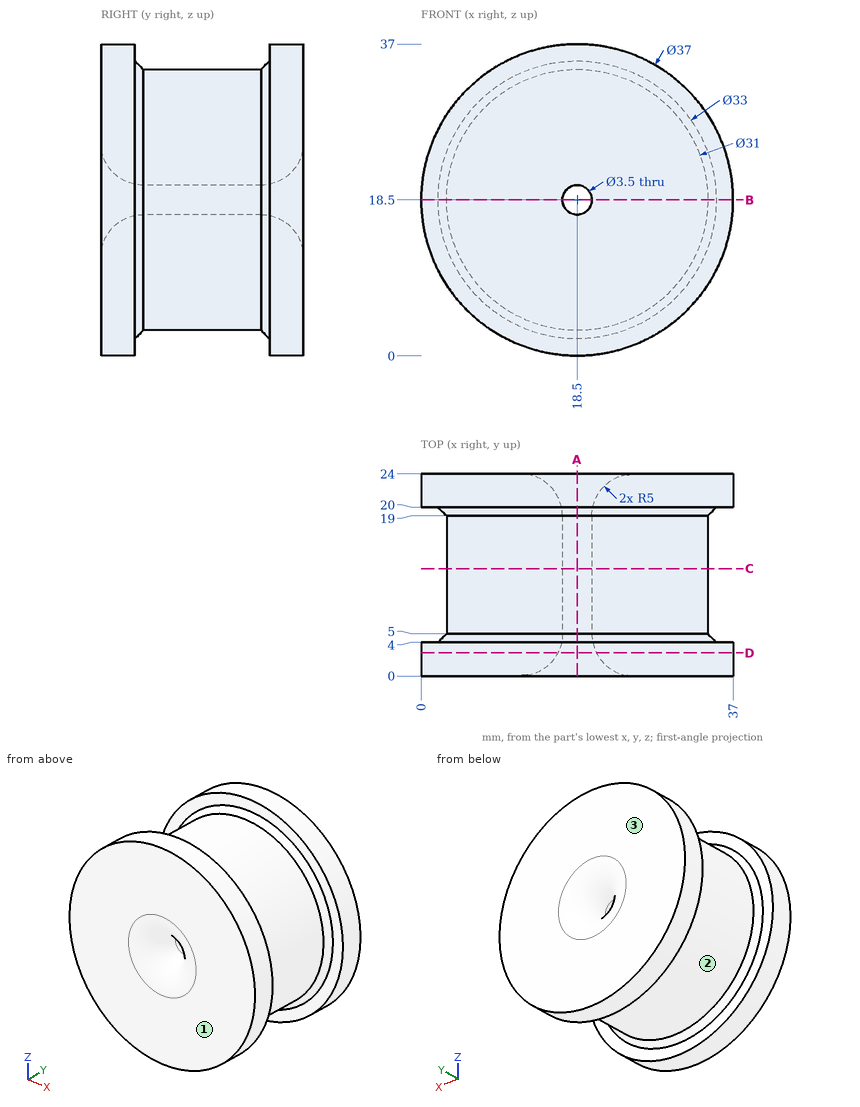
Study the drawing (mm; zero at the part's minimum x, y, z) and answer. Round coordinates to 2 decimals unless told otherwise and drop trailing zeros. Order: outer loops, then holes, each group sorted by start corner. A loop starts at its lowest first (then second) coordinate and runs counter-clockwise, first axis right, second up. Notation, with made-up numbers: (-33.75, -16) - (10.25, -16) arc R16 cw to (10.25, 12) - close; hole circle Ø6 at (83.5, 66.5). An arc over 180 degrees is marked (long way). Use one line per item in the form item = value. Start each with the question number.
(1) Find the intervals of material crossed by line 1 along X through (y, z) = (9, 18.5); line 2 along Y through (x, z) = (21, 12.5); line 3 along Y through (x, z) = (21, 2), in increasing order. Write a range as from..to.
(2) Flat-ended cylindrical pins translate along their axes: pin 1 Ø8 at (y, z) = (14.5, 7) entering from +X; pin 2 Ø8 at (x, y) = (29, 12) entering from +Z; pin 3 Ø12 at (y, z) = (18.5, 8) entering from +X; pin 4 Ø3 at (x, z) = (18.5, 18.5) entering from +Y. Find the tip coordinate at first contact, or state that the pin passes through.
(3) The part is cut by section B-B (z = 18.5). Give the vertices of the cut face in (x, y).
(4) The part is cut by section D-D (y = 2.75). Give the vertices of the cut face in (x, z).
(5) The part is cut by section A-A (x = 18.5). Give the vertices of the cut face in (y, z).
(6) Determine the mould class of the marked faces 1, 2 and 3 for opening direction Y: +Y half, -Y half, draft (parallel to the pull), parting line (faces both ways), or undercut.
(7) The part is cut by section C-C (y = 12.75). Give the vertices of the cut face in (x, z).
Checked values:
q1.line_1 = 3..16.75, 20.25..34
q1.line_2 = 0.01..23.99
q1.line_3 = 0..4, 20..24
q2.pin_1 = 32.06
q2.pin_2 = 32.57
q2.pin_3 = 36.4
q2.pin_4 = through
q3.outline = (0, 0) - (11.75, 0) arc R5 ccw to (16.75, 5) - (16.75, 19) arc R5 ccw to (11.75, 24) - (0, 24) - (0, 20) - (2, 20) - (3, 19) - (3, 5) - (2, 4) - (0, 4) - close; (20.25, 5) arc R5 ccw to (25.25, 0) - (37, 0) - (37, 4) - (35, 4) - (34, 5) - (34, 19) - (35, 20) - (37, 20) - (37, 24) - (25.25, 24) arc R5 ccw to (20.25, 19) - close
q4.outline = circle Ø37 at (18.5, 18.5); hole circle Ø4.57 at (18.5, 18.5)
q5.outline = (0, 0) - (4, 0) - (4, 2) - (5, 3) - (19, 3) - (20, 2) - (20, 0) - (24, 0) - (24, 11.75) arc R5 ccw to (19, 16.75) - (5, 16.75) arc R5 ccw to (0, 11.75) - close; (0, 25.25) arc R5 ccw to (5, 20.25) - (19, 20.25) arc R5 ccw to (24, 25.25) - (24, 37) - (20, 37) - (20, 35) - (19, 34) - (5, 34) - (4, 35) - (4, 37) - (0, 37) - close
q6.face_1 = -Y half
q6.face_2 = undercut
q6.face_3 = +Y half
q7.outline = circle Ø31 at (18.5, 18.5); hole circle Ø3.5 at (18.5, 18.5)
